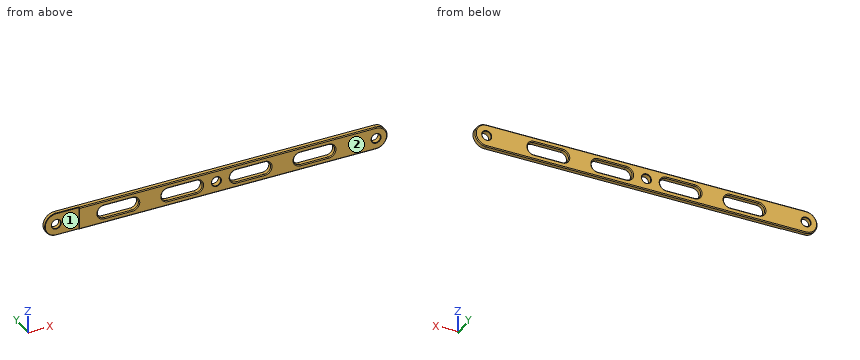
from build123d import *

# Parameters (mm, degrees)
ESQUISSE1_R             = 5
BOSS_EXTRU_1_DEPTH      = 6
ESQUISSE2_R             = 5
ENL_V_MAT_EXTRU_1_DEPTH = 1
CHANFREIN7_SIZE         = 0.5
CHANFREIN8_SIZE         = 1
CHANFREIN9_SIZE         = 1
CHANFREIN10_SIZE        = 1
CHANFREIN11_SIZE        = 0.5
CHANFREIN12_SIZE        = 0.5


with BuildPart() as part:
    # Esquisse1 → Boss.-Extru.1 (new body)
    with BuildSketch(Plane(origin=(0, 0, 0), x_dir=(1, 0, 0), z_dir=(0, 1, 0))):
        with BuildLine():
            Line((0, 12.5), (350, 12.5))
            ThreePointArc((350, 12.5), (362.5, 0), (350, -12.5))
            Line((350, -12.5), (0, -12.5))
            ThreePointArc((0, -12.5), (-12.5, 0), (0, 12.5))
        make_face()
        with Locations(Location((0, 0, 0), (0, 0, 270))):  # turned: the seam where the file's is
            Circle(ESQUISSE1_R, mode=Mode.SUBTRACT)
        with Locations(Location((350, 0, 0), (0, 0, 270))):  # turned: the seam where the file's is
            Circle(ESQUISSE1_R, mode=Mode.SUBTRACT)
        with Locations(Location((175, 0, 0), (0, 0, 270))):  # turned: the seam where the file's is
            Circle(ESQUISSE1_R, mode=Mode.SUBTRACT)
        with BuildLine():
            Line((52, 7), (83, 7))
            ThreePointArc((83, 7), (90, 0), (83, -7))
            Line((83, -7), (52, -7))
            ThreePointArc((52, -7), (45, 0), (52, 7))
        make_face(mode=Mode.SUBTRACT)
        with BuildLine():
            Line((122, 7), (153, 7))
            ThreePointArc((153, 7), (160, 0), (153, -7))
            Line((153, -7), (122, -7))
            ThreePointArc((122, -7), (115, 0), (122, 7))
        make_face(mode=Mode.SUBTRACT)
        with BuildLine():
            Line((197, 7), (228, 7))
            ThreePointArc((228, 7), (235, 0), (228, -7))
            Line((228, -7), (197, -7))
            ThreePointArc((197, -7), (190, 0), (197, 7))
        make_face(mode=Mode.SUBTRACT)
        with BuildLine():
            Line((267, 7), (298, 7))
            ThreePointArc((298, 7), (305, 0), (298, -7))
            Line((298, -7), (267, -7))
            ThreePointArc((267, -7), (260, 0), (267, 7))
        make_face(mode=Mode.SUBTRACT)
    extrude(amount=BOSS_EXTRU_1_DEPTH)

    # Esquisse2 → Enlèv. mat.-Extru.1 (cut)
    with BuildSketch(Plane.XZ):
        with BuildLine():
            Line((0, -12.5), (25, -12.5))
            Line((25, -12.5), (25, 12.5))
            Line((25, 12.5), (0, 12.5))
            ThreePointArc((0, 12.5), (-12.5, 0), (0, -12.5))
        make_face()
        with Locations(Location((0, 0, 0), (0, 0, 270))):  # turned: the seam where the file's is
            Circle(ESQUISSE2_R, mode=Mode.SUBTRACT)
    extrude(amount=-ENL_V_MAT_EXTRU_1_DEPTH, mode=Mode.SUBTRACT)

    # Chanfrein7
    chanfrein7_edges = [part.edges().sort_by_distance(p)[0] for p in [
        (-12.5, 1, 0),
        (12.5, 1, 12.5),
        (12.5, 1, -12.5),
    ]]
    chamfer(chanfrein7_edges, length=CHANFREIN7_SIZE)

    # Chanfrein8
    chanfrein8_edges = [part.edges().sort_by_distance(p)[0] for p in [
        (190, 0, 0),
        (212.5, 0, 7),
        (235, 0, 0),
        (212.5, 0, -7),
        (190, 6, 0),
        (212.5, 6, 7),
        (235, 6, 0),
        (212.5, 6, -7),
        (45, 0, 0),
        (67.5, 0, 7),
        (90, 0, 0),
        (67.5, 0, -7),
        (45, 6, 0),
        (67.5, 6, 7),
        (90, 6, 0),
        (67.5, 6, -7),
        (160, 0, 0),
        (137.5, 0, -7),
        (115, 0, 0),
        (137.5, 0, 7),
        (160, 6, 0),
        (137.5, 6, -7),
        (115, 6, 0),
        (137.5, 6, 7),
        (305, 0, 0),
        (282.5, 0, -7),
        (260, 0, 0),
        (282.5, 0, 7),
        (305, 6, 0),
        (282.5, 6, -7),
        (260, 6, 0),
        (282.5, 6, 7),
    ]]
    chamfer(chanfrein8_edges, length=CHANFREIN8_SIZE)

    # Chanfrein9
    chanfrein9_edges = [part.edges().sort_by_distance(p)[0] for p in [
        (187.5, 0, -12.5),
        (362.5, 0, 0),
        (187.5, 0, 12.5),
    ]]
    chamfer(chanfrein9_edges, length=CHANFREIN9_SIZE)

    # Chanfrein10
    chanfrein10_edges = [part.edges().sort_by_distance(p)[0] for p in [
        (362.5, 6, 0),
        (175, 6, -12.5),
        (-12.5, 6, 0),
        (175, 6, 12.5),
    ]]
    chamfer(chanfrein10_edges, length=CHANFREIN10_SIZE)

    # Chanfrein11
    chanfrein11_edges = [part.edges().sort_by_distance(p)[0] for p in [
        (175, 0, -5),
        (175, 6, -5),
    ]]
    chamfer(chanfrein11_edges, length=CHANFREIN11_SIZE)

    # Chanfrein12
    chanfrein12_edges = [part.edges().sort_by_distance(p)[0] for p in [
        (350, 0, -5),
        (350, 6, -5),
        (0, 6, -5),
        (0, 1, -5),
    ]]
    chamfer(chanfrein12_edges, length=CHANFREIN12_SIZE)


solid = part.part
CAD build for the part. Positions are in the model's coordinates, mm. Face numbers are marked on the shaded views. A direction names the side the tool comes from. Round coordinates to 2 decimals unless told otherwise and drop trailing zeros. Loops run counter-clockwise (first coordinate to the right, second up) from the corner with the lowest first, then second, coordinate; pieces in that order, holes last. Notation, with made-up numbers: (8.25, 64.5) - (60.25, 64.5) arc R24 cw to (60.25, 88.5) - close; hole circle Ø6 at (79, 27.5). An arc over 180 degrees is marked (long way). Put each result on its own line as item: value.
1. Slice it at B-B on y = 3. List the corners of the cut face in (x, z).
Geometry check:
outline: (0, -12.5) - (350, -12.5) arc R12.5 ccw to (350, 12.5) - (0, 12.5) arc R12.5 ccw to start; hole circle Ø10 at (0, 0); hole (52, -7) - (83, -7) arc R7 ccw to (83, 7) - (52, 7) arc R7 ccw to start; hole (122, -7) - (153, -7) arc R7 ccw to (153, 7) - (122, 7) arc R7 ccw to start; hole circle Ø10 at (175, 0); hole (197, -7) - (228, -7) arc R7 ccw to (228, 7) - (197, 7) arc R7 ccw to start; hole (267, -7) - (298, -7) arc R7 ccw to (298, 7) - (267, 7) arc R7 ccw to start; hole circle Ø10 at (350, 0)
2. 3-axis set-ups, long thin cutter, end or side, ignore diameter. For the marked faces 1 and 2: which of +Z, -Z, +X, -X, +Y, -Y reach the whole face in a straight line?
Geometry check:
face 1: +Z, -Z, -X, -Y
face 2: +Z, -Z, +X, -X, -Y
3. Wall check: line 1 (Z direction, x = 211.5, y = 2); line 2 (Z direction, x = 350, y = 3.6); line 3 (Z direction, x = 163, y = 5.25). Give the ranges that are in metal, low to high.
Geometry check:
line 1: -12.5 to -7, 7 to 12.5
line 2: -12.5 to -5, 5 to 12.5
line 3: -12.25 to 12.25
4. Pin check, flat tips, straight feed: P1, Ø0.5, axis at y = 1, z = 5, coming from the -X side; P2, Ø13, axis at x = 0, z = 0, coming from the -Y side. Stop position of each tip, or through.
Geometry check:
P1: x = -11.2
P2: y = 1
5. Slice it at A-A on x = 175. List the corners of the cut face in (y, z), and give its area (3 significant figures).
Geometry check:
outline: (0, -11.5) - (1, -12.5) - (5, -12.5) - (6, -11.5) - (6, -5.5) - (5.5, -5) - (0.5, -5) - (0, -5.5) - close; (0, 5.5) - (0.5, 5) - (5.5, 5) - (6, 5.5) - (6, 11.5) - (5, 12.5) - (1, 12.5) - (0, 11.5) - close
area: 87.5 mm²
